from build123d import *

# Parameters (mm, degrees)
F0_R     = 2.5
F1_DEPTH = 5


with BuildPart() as f1:
    # F0 (on Front) → F1 (new body)
    with BuildSketch(Plane.XZ):
        with BuildLine():
            Line((49, 4), (0, 4))
            ThreePointArc((0, 4), (-2.59533, 3.043725), (-3.949735, 0.632132))
            Line((-3.949735, 0.632132), (-9.749735, -35.607868))
            ThreePointArc((-9.749735, -35.607868), (-6.432132, -40.189735), (-1.850265, -36.872132))
            Line((-1.850265, -36.872132), (-0.631829, -29.25901))
            ThreePointArc((-0.631829, -29.25901), (9.526214, -11.17206), (28.991186, -4))
            Line((28.991186, -4), (49, -4))
            ThreePointArc((49, -4), (53, 0), (49, 4))
        make_face()
        with Locations((-5.8, -36.24)):
            Circle(F0_R, mode=Mode.SUBTRACT)
        Circle(F0_R, mode=Mode.SUBTRACT)
        with Locations((49, 0)):
            Circle(F0_R, mode=Mode.SUBTRACT)
    extrude(amount=F1_DEPTH)


solid = f1.part
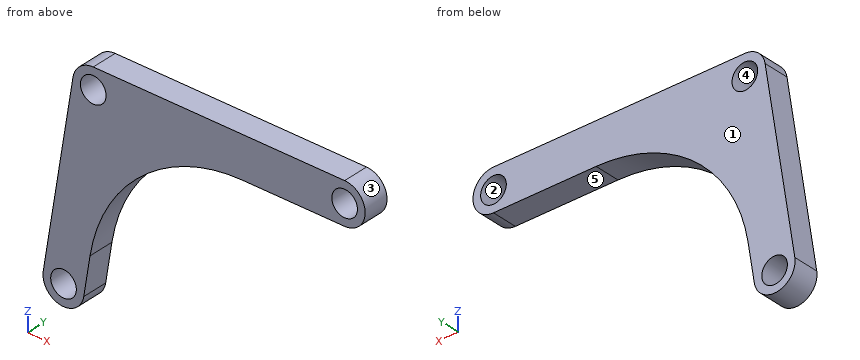
Geometry check sheet. Reference: the model listing, model coordinates, mm. Face numbers are marked on the shaded views. A direction names the side the tool comes from. Give positions to 0.01 mm unless a question says otherwise; leave off trailing zeros. Loops run counter-clockwise (first coordinate to the right, second up) from the corner with the lowest first, then second, coordinate; pieces in that order, holes last.
(1) Section check D-D on x = 30. Record the cut outline in (y, z).
From the geometry:
outline: (-5, -4) - (0, -4) - (0, 4) - (-5, 4) - close
(2) Section check A-A on y = -1.45. Record the cut outline in (x, z), then the cut area to 3 significant figures.
From the geometry:
outline: (-9.75, -35.61) arc R4 ccw to (-1.85, -36.87) - (-0.63, -29.26) arc R30 cw to (28.99, -4) - (49, -4) arc R4 ccw to (49, 4) - (0, 4) arc R4 ccw to (-3.95, 0.63) - close; hole circle Ø5 at (-5.8, -36.24); hole circle Ø5 at (0, 0); hole circle Ø5 at (49, 0)
area: 807 mm2
(3) Depth check by flat-ended pin: pin 1 Ø2 at (x, y) = (2.5, -3.5) entering from -Z; pin 2 Ø1.5 at (y, z) = (-1, -27.5) entering from -X. Enter the tip coordinate at first touch or a pass-through.
From the geometry:
pin 1: stops at z = -21.99
pin 2: stops at x = -8.57
(4) Set-up check for the marked faces 4 and 5: record each of +Z, -Z, +X, -X, +Y, -Y from which the full face is reachable in a straight line by a thin tool's end or side.
From the geometry:
face 4: +Y, -Y
face 5: -Z, +X, +Y, -Y
(5) Section check B-B on z = 0. Record the cut outline in (x, y).
From the geometry:
outline: (-4.05, -5) - (-2.5, -5) - (-2.5, 0) - (-4.05, 0) - close; (2.5, -5) - (46.5, -5) - (46.5, 0) - (2.5, 0) - close; (51.5, -5) - (53, -5) - (53, 0) - (51.5, 0) - close
(6) Thickness scan on L1, parallel to Z at x = 49, y = -3.2; L2, parallel to X at y = -3.15, z = -1; L3, parallel to X at y = -3.6, z = 1.5. Record the ranges inside material, lowest first.
From the geometry:
L1: z = -4 to -2.5, 2.5 to 4
L2: x = -4.21 to -2.29, 2.29 to 46.71, 51.29 to 52.87
L3: x = -3.71 to -2, 2 to 47, 51 to 52.71
(7) Section check C-C on x = -5.8. Record the cut outline in (y, z).
From the geometry:
outline: (-5, -40.24) - (0, -40.24) - (0, -38.74) - (-5, -38.74) - close; (-5, -33.74) - (0, -33.74) - (0, -10.93) - (-5, -10.93) - close
(8) Release check for a two-part mould opening along Z. For the marked faces 1, 2 and 3 record: released by +Z, released by -Z, zero draft, split by the parting line, or undercut.
From the geometry:
face 1: zero draft
face 2: undercut
face 3: split by the parting line
